from build123d import *

# Parameters (mm, degrees)
SKETCH1_W           = 20
SKETCH1_H           = 17
BOSS_EXTRUDE1_DEPTH = 1
SKETCH2_R           = 1.6
SKETCH2_R_2         = 1
BOSS_EXTRUDE2_DEPTH = 20
FILLET1_R           = 10
FILLET2_R           = 0.5
SKETCH4_W           = 10
SKETCH4_H           = 10.104734337
CUT_EXTRUDE3_DEPTH  = 15.86420015


with BuildPart() as part:
    # Sketch1 → Boss-Extrude1 (new body)
    with BuildSketch(Plane(origin=(0, 0, 0), x_dir=(1, 0, 0), z_dir=(0, 1, 0))):
        Rectangle(SKETCH1_W, SKETCH1_H)
    extrude(amount=BOSS_EXTRUDE1_DEPTH)

    # Sketch2 → Boss-Extrude2 (add)
    with BuildSketch(Plane(origin=(10, 0, 0), x_dir=(0, 0, -1), z_dir=(1, 0, 0))):
        with Locations((8.800384095, 1.974416987)):
            Circle(SKETCH2_R)
        with Locations((8.800384095, 1.974416987)):
            Circle(SKETCH2_R_2, mode=Mode.SUBTRACT)
    extrude(amount=-BOSS_EXTRUDE2_DEPTH)

    # Fillet1
    # the kernel refuses this fillet: 10 mm, written as the material it adds along each edge
    with BuildSketch(Plane(origin=(-10, 0.402866989, -8.5), x_dir=(0, -1, 0), z_dir=(1, 0, 0))) as fillet1_piece_1:
        with BuildLine():
            CenterArc((8.937605274, 5.21135706), FILLET1_R, 205.046884286, 6.361578996)
            Line((-0.12201134, 0.977759676), (-0.303203672, 0.893087728))
            ThreePointArc((-0.303203672, 0.893087728), (-0.18232452, 0.473740867), (-0.19644375, 0.037548012))
            Line((-0.19644375, 0.037548012), (0, -0.2))
            ThreePointArc((0, -0.2), (0.201433495, -0.2), (0.232172223, -0.104227141))
            Line((0.232172223, -0.104227141), (0.402866989, 0))
        make_face()
    extrude(amount=20)

    # Fillet2
    fillet2_edges = [part.edges().sort_by_distance(p)[0] for p in [
        (0, 0, -8.5),
    ]]
    fillet(fillet2_edges, radius=FILLET2_R)

    # Sketch4 → Cut-Extrude3 (cut, through all)
    with BuildSketch(Plane(origin=(0, 0, 0), x_dir=(1, 0, 0), z_dir=(0, 1, 0))):
        with Locations((0, 11.80749184)):
            Rectangle(SKETCH4_W, SKETCH4_H)
    extrude(amount=CUT_EXTRUDE3_DEPTH, mode=Mode.SUBTRACT)


solid = part.part
Geometry check sheet. Reference: the model listing, model coordinates, mm. A direction names the side the tool comes from. Round coordinates to 2 decimals unless told otherwise and drop trailing zeros. Write each loop counter-clockwise with the first axis right and the second up, starting at its lowest first coordinate (ties: lowest second). Pieces come first, ordered by that corner, then holes. Notation, with made-up numbers: (-2.5, 33) -> (53.5, 33) arc R32 ccw to (53.5, 64) -> close; hole circle Ø3 at (8, -40). An arc over 180 degrees is marked (long way). One line per item, written item: value. Start each with the question number.
(1) Cross-section at B-B, the plane y = 1.5. Record the cut outline in (x, z).
(2) Draft check along Y on faces 3 (the cylindrical face through (7.465, 0.311, -9.047)), 4 (the cylindrical face through (-7.465, 1.591, -9.724)), 5 (the flat face through (-0.1, 0.5, -6.755)), 6 (the cylindrical face through (7.535, 1.591, -9.724)). Enter one of: +Y half, -Y half, draft (parallel to the pull), parting line (faces both ways), or undercut.
(3) Scan lines: line 1 (X direction, y = 3, z = -8.25); line 2 (Y direction, x = -1, z = 0); line 3 (Z direction, x = 3.75, y = 0.95). Record each from-to range of solid material in increasing order. Write a range as [from, to].
(4) Go/stop test with flat-tipped pins: pin 1 Ø4 at (x, z) = (6.5, 3) entering from +Y; pin 2 Ø0.5 at (x, y) = (-0.5, 0.5) entering from -Z; pin 3 Ø6 at (x, z) = (-4, -5.5) entering from +Y; pin 4 Ø1.2 at (y, z) = (1.97, -8.8) entering from -X. Record where each tip stops, or that it passes through.
(5) Cross-section at C-C, the plane x = 7. Record the cut outline in (y, z), and give its area (3 significant figures).
(6) Access from +Z, -Z, +X, -X, +Y, -Y to the whole of each face (thin tool, end or side, straight path). Record for faces 1 (the flat face through (5, 1, -8)), 2 (the flat face through (-10, 0.6, -1.1)).
(7) Cross-section at A-A, the plane z = -9. Record the cut outline in (x, y).
(8) Cross-section at D-D, the plane z = 1. Record the cut outline in (x, y).
Answer:
1. outline: (-10, -10.33) -> (-5, -10.33) -> (-5, -9.68) -> (-10, -9.68) -> close; (-10, -7.92) -> (-5, -7.92) -> (-5, -7.27) -> (-10, -7.27) -> close; (5, -10.33) -> (10, -10.33) -> (10, -9.68) -> (5, -9.68) -> close; (5, -7.92) -> (10, -7.92) -> (10, -7.27) -> (5, -7.27) -> close
2. face 3: -Y half
2. face 4: undercut
2. face 5: draft
2. face 6: undercut
3. line 1: [-10, -5], [5, 10]
3. line 2: [0, 1]
3. line 3: [-6.76, 8.5]
4. pin 1: y = 1
4. pin 2: z = -6.76
4. pin 3: y = 3.5
4. pin 4: through
5. outline: (0, -8.36) arc R0.5 ccw to (0.07, -8.62) arc R10 cw to (0.52, -9.48) arc R1.6 ccw (long way) to (1, -7.53) -> (1, 8.5) -> (0, 8.5) -> close; hole circle Ø2 at (1.97, -8.8)
5. area: 21.7 mm²
6. face 1: -Z, +Y, -Y
6. face 2: +Z, -Z, -X, +Y, -Y
7. outline: (-10, 0.29) -> (-5, 0.29) -> (-5, 0.99) -> (-10, 0.99) -> close; (-10, 2.95) -> (-5, 2.95) -> (-5, 3.56) -> (-10, 3.56) -> close; (5, 0.29) -> (10, 0.29) -> (10, 0.99) -> (5, 0.99) -> close; (5, 2.95) -> (10, 2.95) -> (10, 3.56) -> (5, 3.56) -> close
8. outline: (-10, 0) -> (10, 0) -> (10, 1) -> (-10, 1) -> close
